Geometry: final body of the model. Coordinates: model frame, mm. Give positions to 0.01 mm unless a question says otherwise; leave off trailing zeros. Loops run counter-clockwise (first coordinate to the right, second up) from the corner with the lowest first, then second, coordinate; pieces in that order, holes last.
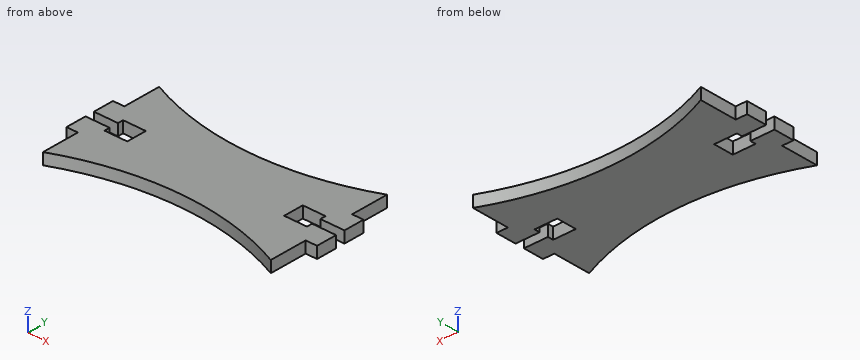
from build123d import *

# Parameters (mm, degrees)
BOSS_EXTRUDE1_DEPTH = 4.5


with BuildPart() as part:
    # Sketch1 → Boss-Extrude1 (new body)
    with BuildSketch(Plane.XY):
        with BuildLine():
            Line((-49.5, -1.8), (-49.5, -10))
            Line((-49.5, -10), (-45, -10))
            Line((-45, -10), (-45, -25))
            ThreePointArc((-45, -25), (0, -15.341439003), (45, -25))
            Line((45, -25), (45, -10))
            Line((45, -10), (49.5, -10))
            Line((49.5, -10), (49.5, -1.8))
            Line((49.5, -1.8), (40, -1.8))
            Line((40, -1.8), (40, -4))
            Line((40, -4), (31, -4))
            Line((31, -4), (31, 4))
            Line((31, 4), (40, 4))
            Line((40, 4), (40, 1.8))
            Line((40, 1.8), (49.5, 1.8))
            Line((49.5, 1.8), (49.5, 10))
            Line((49.5, 10), (45, 10))
            Line((45, 10), (45, 25))
            ThreePointArc((45, 25), (0, 15.341439003), (-45, 25))
            Line((-45, 25), (-45, 10))
            Line((-45, 10), (-49.5, 10))
            Line((-49.5, 10), (-49.5, 1.8))
            Line((-49.5, 1.8), (-40, 1.8))
            Line((-40, 1.8), (-40, 4))
            Line((-40, 4), (-31, 4))
            Line((-31, 4), (-31, -4))
            Line((-31, -4), (-40, -4))
            Line((-40, -4), (-40, -1.8))
            Line((-40, -1.8), (-49.5, -1.8))
        make_face()
    extrude(amount=BOSS_EXTRUDE1_DEPTH)


solid = part.part
Item 1: Section query C-C on z = 3. Return loops of the section in (x, y), plus the area to 3 significant figures.
Values follow:
outline: (-49.5, -10) - (-45, -10) - (-45, -25) arc R109.66 cw to (45, -25) - (45, -10) - (49.5, -10) - (49.5, -1.8) - (40, -1.8) - (40, -4) - (31, -4) - (31, 4) - (40, 4) - (40, 1.8) - (49.5, 1.8) - (49.5, 10) - (45, 10) - (45, 25) arc R109.66 cw to (-45, 25) - (-45, 10) - (-49.5, 10) - (-49.5, 1.8) - (-40, 1.8) - (-40, 4) - (-31, 4) - (-31, -4) - (-40, -4) - (-40, -1.8) - (-49.5, -1.8) - close
area: 3,300 mm2
Item 2: Section query D-D on x = 25.5. Return loops of the section in (y, z).
Values follow:
outline: (-18.35, 0) - (18.35, 0) - (18.35, 4.5) - (-18.35, 4.5) - close
Item 3: Ray query, probe 1 along X at (y, z) = (-2.5, 0.5); probe 2 along X at (y, z) = (-12.5, 1.85); probe 3 along Y at (x, z) = (-35.5, 3.35). Return the intervals inside material, ascending.
Values follow:
probe 1: x = -49.5 to -40, -31 to 31, 40 to 49.5
probe 2: x = -45 to 45
probe 3: y = -21.25 to -4, 4 to 21.25
Item 4: Section query A-A on y = -17. Return loops of the section in (x, z), plus the area to 3 significant figures.
Values follow:
outline: (-45, 0) - (-19, 0) - (-19, 4.5) - (-45, 4.5) - close; (19, 0) - (45, 0) - (45, 4.5) - (19, 4.5) - close
area: 234 mm2
Item 5: Section query B-B on x = 41. Return loops of the section in (y, z), plus the area to 3 significant figures.
Values follow:
outline: (-23.29, 0) - (-1.8, 0) - (-1.8, 4.5) - (-23.29, 4.5) - close; (1.8, 0) - (23.29, 0) - (23.29, 4.5) - (1.8, 4.5) - close
area: 193 mm2
Item 6: Pin query (flat end, axial travel): pin 1 (1.3 mm diameter, centred on y = -1, z = 1.5, fed in from -X); pin 2 (1.3 mm diameter, centred on x = -35, z = 1.5, fed in from -Y). Return the tip coordinate at first contact, or that it passes through.
Values follow:
pin 1: stops at x = -31
pin 2: stops at y = -21.3
